from build123d import *

# Parameters (mm, degrees)
SKETCH_1_R           = 1.1
SKETCH_1_R_2         = 4
EXTRUDE_1_DEPTH      = 2.5
SKETCH_2_W           = 14.4
SKETCH_2_H           = 0.5
CUT_EXTRUDE_1_DEPTH  = 37.005863078
SKETCH_3_W           = 13
SKETCH_3_H           = 1.3
CUT_EXTRUDE_2_DEPTH  = 4.5
SKETCH_4_W           = 13
SKETCH_4_H           = 1.3
CUT_EXTRUDE_3_DEPTH  = 4.5
SKETCH_5_W           = 11.5
SKETCH_5_H           = 17.3
CUT_EXTRUDE_11_DEPTH = 0.5
SKETCH_6_W           = 6
SKETCH_6_H           = 10
CUT_EXTRUDE_12_DEPTH = 0.5
FILLET_1_R           = 0.5
FILLET_2_R           = 1
SKETCH_7_W           = 4.3
SKETCH_7_H           = 13.3
CUT_EXTRUDE_13_DEPTH = 30.401057536
CHAMFER_1_SIZE       = 0.699461487
CHAMFER_1_SIZE_2     = 1.5


with BuildPart() as part:
    # 草图1 → 凸台-拉伸1 (new body)
    with BuildSketch(Plane(origin=(0, 0, 0), x_dir=(1, 0, 0), z_dir=(0, 1, 0))):
        with BuildLine():
            Line((-12, 24.224), (-12, -10.776))
            ThreePointArc((-12, -10.776), (-11.267766953, -12.543766953), (-9.5, -13.276))
            Line((-9.5, -13.276), (9.5, -13.276))
            ThreePointArc((9.5, -13.276), (11.267766953, -12.543766953), (12, -10.776))
            Line((12, -10.776), (12, 24.224))
            ThreePointArc((12, 24.224), (11.267766953, 25.991766953), (9.5, 26.724))
            Line((9.5, 26.724), (-9.5, 26.724))
            ThreePointArc((-9.5, 26.724), (-11.267766953, 25.991766953), (-12, 24.224))
        make_face()
        with Locations(Location((-9.714, -10.986, 0), (0, 0, 270))):
            Circle(SKETCH_1_R, mode=Mode.SUBTRACT)
        with Locations(Location((0, 0.32, 0), (0, 0, 270))):
            Circle(SKETCH_1_R_2, mode=Mode.SUBTRACT)
        with Locations(Location((9.714, -10.986, 0), (0, 0, 270))):
            Circle(SKETCH_1_R, mode=Mode.SUBTRACT)
        with Locations(Location((9.714, 10.986, 0), (0, 0, 270))):
            Circle(SKETCH_1_R, mode=Mode.SUBTRACT)
        with Locations(Location((-9.714, 10.986, 0), (0, 0, 270))):
            Circle(SKETCH_1_R, mode=Mode.SUBTRACT)
    extrude(amount=-EXTRUDE_1_DEPTH)

    # 草图2 → 切除-拉伸1 (cut, through all)
    with BuildSketch(Plane(origin=(12, 0, 0), x_dir=(0, 0, -1), z_dir=(1, 0, 0))):
        with Locations((0.924, -2.25)):
            Rectangle(SKETCH_2_W, SKETCH_2_H)
    extrude(amount=-CUT_EXTRUDE_1_DEPTH, mode=Mode.SUBTRACT)

    # 草图3 → 切除-拉伸2 (cut)
    with BuildSketch(Plane(origin=(12, 0, 0), x_dir=(0, 0, -1), z_dir=(1, 0, 0))):
        with Locations((1.624, -1.85)):
            Rectangle(SKETCH_3_W, SKETCH_3_H)
    extrude(amount=-CUT_EXTRUDE_2_DEPTH, mode=Mode.SUBTRACT)

    # 草图4 → 切除-拉伸3 (cut)
    with BuildSketch(Plane.ZY.offset(12)):
        with Locations((-1.624, -1.85)):
            Rectangle(SKETCH_4_W, SKETCH_4_H)
    extrude(amount=-CUT_EXTRUDE_3_DEPTH, mode=Mode.SUBTRACT)

    # 草图5 → 切除-拉伸11 (cut)
    with BuildSketch(Plane.XZ.offset(2.5)):
        with Locations((1.75, -16.774)):
            Rectangle(SKETCH_5_W, SKETCH_5_H)
    extrude(amount=-CUT_EXTRUDE_11_DEPTH, mode=Mode.SUBTRACT)

    # 草图6 → 切除-拉伸12 (cut)
    with BuildSketch(Plane.XZ.offset(2)):
        with Locations((-1, -13.124)):
            Rectangle(SKETCH_6_W, SKETCH_6_H)
    extrude(amount=-CUT_EXTRUDE_12_DEPTH, mode=Mode.SUBTRACT)

    # 圆角1
    # the kernel refuses this fillet: 0.5 mm, written as the material it takes off along each edge
    with BuildSketch(Plane(origin=(-9.5, 0, 13.276), x_dir=(0, 0, -1), z_dir=(1, 0, 0))) as fillet_1_piece_1:
        with BuildLine():
            CenterArc((FILLET_1_R, -FILLET_1_R), FILLET_1_R, 90, 90)
            Line((0, -FILLET_1_R), (-FILLET_1_R * 0.02, -FILLET_1_R))
            Line((-FILLET_1_R * 0.02, -FILLET_1_R), (-FILLET_1_R * 0.02, FILLET_1_R * 0.02))
            Line((-FILLET_1_R * 0.02, FILLET_1_R * 0.02), (FILLET_1_R, FILLET_1_R * 0.02))
            Line((FILLET_1_R, FILLET_1_R * 0.02), (FILLET_1_R, 0))
        make_face()
    extrude(amount=19, mode=Mode.SUBTRACT)
    with BuildSketch(Plane(origin=(-9.5, 0, 10.776), x_dir=(-1, 0, 0), z_dir=(0, 0, -1))) as fillet_1_piece_2:
        with BuildLine():
            CenterArc((2.5 - FILLET_1_R, -FILLET_1_R), FILLET_1_R, 0, 90)
            Line((2.5, -FILLET_1_R), (2.5 + FILLET_1_R * 0.02, -FILLET_1_R))
            Line((2.5 + FILLET_1_R * 0.02, -FILLET_1_R), (2.5 + FILLET_1_R * 0.02, FILLET_1_R * 0.02))
            Line((2.5 + FILLET_1_R * 0.02, FILLET_1_R * 0.02), (2.5 - FILLET_1_R, FILLET_1_R * 0.02))
            Line((2.5 - FILLET_1_R, FILLET_1_R * 0.02), (2.5 - FILLET_1_R, 0))
        make_face()
    revolve(axis=Axis((-9.5, 0, 10.776), (0, 1, 0)), revolution_arc=90, mode=Mode.SUBTRACT)
    with BuildSketch(Plane(origin=(-12, 0, -27.224), x_dir=(0, -1, 0), z_dir=(0, 0, 1))) as fillet_1_piece_3:
        with BuildLine():
            CenterArc((FILLET_1_R, FILLET_1_R), FILLET_1_R, 180, 90)
            Line((0, FILLET_1_R), (-FILLET_1_R * 0.02, FILLET_1_R))
            Line((-FILLET_1_R * 0.02, FILLET_1_R), (-FILLET_1_R * 0.02, -FILLET_1_R * 0.02))
            Line((-FILLET_1_R * 0.02, -FILLET_1_R * 0.02), (FILLET_1_R, -FILLET_1_R * 0.02))
            Line((FILLET_1_R, -FILLET_1_R * 0.02), (FILLET_1_R, 0))
        make_face()
    extrude(amount=38, mode=Mode.SUBTRACT)
    with BuildSketch(Plane(origin=(12, 0, 10.776), x_dir=(-1, 0, 0), z_dir=(0, 0, -1))) as fillet_1_piece_4:
        with BuildLine():
            CenterArc((FILLET_1_R, -FILLET_1_R), FILLET_1_R, 90, 90)
            Line((0, -FILLET_1_R), (-FILLET_1_R * 0.02, -FILLET_1_R))
            Line((-FILLET_1_R * 0.02, -FILLET_1_R), (-FILLET_1_R * 0.02, FILLET_1_R * 0.02))
            Line((-FILLET_1_R * 0.02, FILLET_1_R * 0.02), (FILLET_1_R, FILLET_1_R * 0.02))
            Line((FILLET_1_R, FILLET_1_R * 0.02), (FILLET_1_R, 0))
        make_face()
    extrude(amount=38, mode=Mode.SUBTRACT)
    with BuildSketch(Plane(origin=(9.5, 0, 10.776), x_dir=(0, 0, 1), z_dir=(-1, 0, 0))) as fillet_1_piece_5:
        with BuildLine():
            CenterArc((2.5 - FILLET_1_R, -FILLET_1_R), FILLET_1_R, 0, 90)
            Line((2.5, -FILLET_1_R), (2.5 + FILLET_1_R * 0.02, -FILLET_1_R))
            Line((2.5 + FILLET_1_R * 0.02, -FILLET_1_R), (2.5 + FILLET_1_R * 0.02, FILLET_1_R * 0.02))
            Line((2.5 + FILLET_1_R * 0.02, FILLET_1_R * 0.02), (2.5 - FILLET_1_R, FILLET_1_R * 0.02))
            Line((2.5 - FILLET_1_R, FILLET_1_R * 0.02), (2.5 - FILLET_1_R, 0))
        make_face()
    revolve(axis=Axis((9.5, 0, 10.776), (0, 1, 0)), revolution_arc=90, mode=Mode.SUBTRACT)

    # 圆角2
    fillet_2_edges = [part.edges().sort_by_distance(p)[0] for p in [
        (0, 0, -4.32),
    ]]
    fillet(fillet_2_edges, radius=FILLET_2_R)

    # 草图7 → 切除-拉伸13 (cut, through all)
    with BuildSketch(Plane(origin=(0, 0, 0), x_dir=(1, 0, 0), z_dir=(0, 1, 0))):
        with Locations((-9.85, 20.074)):
            Rectangle(SKETCH_7_W, SKETCH_7_H)
    extrude(amount=-CUT_EXTRUDE_13_DEPTH, mode=Mode.SUBTRACT)

    # 倒角1
    # the kernel refuses this chamfer: 1.5, 0.699461487 mm, written as the material it takes off along each edge
    with BuildSketch(Plane(origin=(-7.7, 0, -13.424), x_dir=(0, 0.07481330637059964, 0.9971975577536774), z_dir=(-1, 0, 0))) as chamfer_1_piece_1:
        Polygon((CHAMFER_1_SIZE * 0.997197558085, -CHAMFER_1_SIZE * 0.0748133063955), (-CHAMFER_1_SIZE_2 * 0.0748133063706, -CHAMFER_1_SIZE_2 * 0.997197557754), (0, 0), align=None)
    extrude(amount=7.686463207, mode=Mode.SUBTRACT)
    with BuildSketch(Plane(origin=(-7.7, 0, -30.610463207), x_dir=(0.9971975577536775, 0.07481330637059957, 0), z_dir=(0, 0, 1))) as chamfer_1_piece_2:
        Polygon((CHAMFER_1_SIZE * 0.997197558085, -CHAMFER_1_SIZE * 0.0748133063955), (-CHAMFER_1_SIZE_2 * 0.0748133063706, -CHAMFER_1_SIZE_2 * 0.997197557754), (0, 0), align=None)
    extrude(amount=17.186463207, mode=Mode.SUBTRACT)
    with BuildSketch(Plane(origin=(-3.813536793, 0, -13.424), x_dir=(0, 0.07481330637059964, 0.9971975577536774), z_dir=(-1, 0, 0))) as chamfer_1_piece_3a_section:
        Polygon((CHAMFER_1_SIZE * 0.997197558085, -CHAMFER_1_SIZE * 0.0748133063955), (-CHAMFER_1_SIZE_2 * 0.0748133063706, -CHAMFER_1_SIZE_2 * 0.997197557754), (0, 0), align=None)
    chamfer_1_piece_3a = extrude(amount=11.572926414, mode=Mode.PRIVATE)
    chamfer_1_piece_3a = split(chamfer_1_piece_3a, bisect_by=Plane(origin=(-7.7, -0.507353362, -13.203429624), z_dir=(1, 0, 0)), keep=Keep.TOP, mode=Mode.PRIVATE)
    with BuildSketch(Plane(origin=(-7.7, 0, -30.610463207), x_dir=(0.9971975577536775, 0.07481330637059957, 0), z_dir=(0, 0, 1))) as chamfer_1_piece_3b_section:
        Polygon((CHAMFER_1_SIZE * 0.997197558085, -CHAMFER_1_SIZE * 0.0748133063955), (-CHAMFER_1_SIZE_2 * 0.0748133063706, -CHAMFER_1_SIZE_2 * 0.997197557754), (0, 0), align=None)
    chamfer_1_piece_3b = extrude(amount=21.072926414, mode=Mode.PRIVATE)
    chamfer_1_piece_3b = split(chamfer_1_piece_3b, bisect_by=Plane(origin=(-7.479429624, -0.507353362, -13.424), z_dir=(0, 0, 1)), keep=Keep.TOP, mode=Mode.PRIVATE)
    chamfer_1_piece_3 = chamfer_1_piece_3a & chamfer_1_piece_3b
    add(chamfer_1_piece_3, mode=Mode.SUBTRACT)


solid = part.part
Could you check a few things on this model? Use its own coordinates, in mm. A direction names the side the tool comes from. Round coordinates to 2 decimals unless told otherwise and drop trailing zeros. Write each loop counter-clockwise with the first axis right and the second up, starting at its lowest first coordinate (ties: lowest second). Pieces come first, ordered by that corner, then holes. Notation, with made-up numbers: (75.5, 71.25) - (87.5, 71.25) arc R21 cw to (87.5, 104.25) - close; hole circle Ø4 at (-10.5, 55). An arc over 180 degrees is marked (long way). Put each result on its own line as item: value. Start each with the question number.
(1) I want a section at D-D, the plane z = -15.5. Please give me the cut outline in (x, y).
(2) I want a section at B-B, the plane x = 0. Please give me the cut outline in (y, z).
(3) For faces 1 (the flat face through (-4, -2, -15)), 2 (the flat face through (-9.47, -0.74, -13.07)), 3 (the flat face through (10, -2, -8.124)), 4 (the flat face through (-10, -2, -13.424)), which set-ups out of +Z, -Z, +X, -X, +Y, -Y let a thin tool reach every point of the face, with its end or its side?
(4) I want a section at A-A, the plane z = -0.32. Please give me the cut outline in (x, y).
(5) Will these pins go through, and if not, where does the flat tip stop? pin 1 (2 mm diameter, centred on x = -9, z = 0, fed in from -Y); pin 2 (0.9 mm diameter, centred on x = -8.5, y = -1.5, fed in from -Z); pin 3 (1.5 mm diameter, centred on x = 1, z = -11, fed in from -Y).
(6) Thinking about a two-plate mould opening in X: for faces 5 (the flat face through (0, -2.5, 10)), 6 (the cylindrical face through (11.25, -1.49, 12.56)), 7 (the flat face through (-1, -1.5, -13)), which applies, released by +X, released by -X, zero draft, split by the parting line, or undercut?
(7) I want a section at C-C, the plane x = -6. Please give me the cut outline in (y, z), plus the area to 3 significant figures.
(8) I need wall thicknesses on probe 1 along X at (y, z) = (-1.7, -16); probe 2 along Y at (x, z) = (2.5, -17); probe 3 along X at (y, z) = (-0.55, 2). Which ranges of each line are inside material? Lowest first, please.
Here are the results:
1. outline: (-7.7, -2.5) - (-4, -2.5) - (-4, -1.5) - (2, -1.5) - (2, -2) - (7.5, -2) - (7.5, -2.5) - (12, -2.5) - (12, -0.5) arc R0.5 ccw to (11.5, 0) - (-7, 0) - (-7.7, -1.5) - close
2. outline: (-2.5, -26.72) - (0, -26.72) - (0, -5.32) arc R1 ccw to (-1, -4.32) - (-2, -4.32) - (-2, -8.12) - (-1.5, -8.12) - (-1.5, -18.12) - (-2, -18.12) - (-2, -25.42) - (-2.5, -25.42) - close; (-2.5, 6.28) - (-2, 6.28) - (-2, 3.68) - (-1, 3.68) arc R1 ccw to (0, 4.68) - (0, 12.78) arc R0.5 ccw to (-0.5, 13.28) - (-2.5, 13.28) - close
3. face 1: -Y
3. face 2: -Z, -X, +Y
3. face 3: +X, -Y
3. face 4: -Z, -X, +Y, -Y
4. outline: (-12, -1.2) - (-7.5, -1.2) - (-7.5, -2) - (-4, -2) - (-4, -1) arc R1 ccw to (-5, 0) - (-11.5, 0) arc R0.5 ccw to (-12, -0.5) - close; (4, -2) - (7.5, -2) - (7.5, -1.2) - (12, -1.2) - (12, -0.5) arc R0.5 ccw to (11.5, 0) - (5, 0) arc R1 ccw to (4, -1) - close
5. pin 1: stops at y = -1.2
5. pin 2: stops at z = -13.42
5. pin 3: stops at y = -1.5
6. face 5: zero draft
6. face 6: released by +X
6. face 7: undercut
7. outline: (-2.5, -26.72) - (0, -26.72) - (0, 12.78) arc R0.5 ccw to (-0.5, 13.28) - (-2.5, 13.28) - (-2.5, 6.28) - (-2, 6.28) - (-2, -8.12) - (-2.5, -8.12) - close
7. area: 92.7 mm^2
8. probe 1: x = -7.7 to -4, 2 to 12
8. probe 2: y = -2 to 0
8. probe 3: x = -12 to -3.39, 3.39 to 12
